Autodesk Inventor part; units mm, degrees
ref_plane "YZ Plane" through (0, 0, 0) normal (1, 0, 0) x (0, 1, 0)
ref_plane "XZ Plane" through (0, 0, 0) normal (0, 1, 0) x (-1, 0, 0)
ref_plane "XY Plane" through (0, 0, 0) normal (0, 0, 1) x (1, 0, 0)
sketch "Sketch1" plane through (0, 0, 0) normal (0, 0, 1) x (1, 0, 0)
  line L0 (2.1516, 4.7552) -> (14.9532, 4.7552)
  line L1 (14.9532, 4.7552) -> (14.9532, -2.1028)
  line L2 (14.9532, -2.1028) -> (2.1516, -2.1028)
  line L3 (2.1516, -2.1028) -> (2.1516, 4.7552)
  point P0 (0, 0)
  dimension "d0" = 12.8016
  dimension "d1" = 6.858
extrude "Extrusion1" add sketch "Sketch1" along normal blind 13.7414
sketch "Sketch2" plane through (0, 0, 13.7414) normal (0, 0, 1) x (1, 0, 0)
  circle A0 centre (8.5524, 1.3262) radius 2.921
  line L0 (14.9532, -2.1028) -> (14.9532, 4.7552)
  line L1 (14.9532, 4.7552) -> (2.1516, 4.7552)
  point P0 (0, 0)
  dimension "d4" = 5.842
  dimension "d5" = 6.4008
  dimension "d6" = 3.429
extrude "Extrusion2" add sketch "Sketch2" along normal blind 8.89
sketch "Sketch3" plane through (8.5524, 1.3262, 22.6314) normal (0, 0, 1) x (1, 0, 0)
  circle A0 centre (0, 0) radius 1.4986
  point P0 (-8.5524, -1.3262)
  dimension "d9" = 2.9972
extrude "Extrusion3" add sketch "Sketch3" along normal blind 9.906
properties part number "Switch"
Geometry: final body of the model. Coordinates: model frame, mm. A direction names the side the tool comes from. Give positions to 0.01 mm unless a question says otherwise; leave off trailing zeros. Write each loop counter-clockwise with the first axis right and the second up, starting at its lowest first coordinate (ties: lowest second). Pieces come first, ordered by that corner, then holes. Notation, with made-up numbers: M 50.5,73 L 109.5,73 A25 ccw 109.5,112 Z; hole C 43.5,-8 d6. An arc over 180 degrees is marked long. Answer in a Markdown table with one row per item. Add a question column.
(1) Section A-A on x = 13.25. Return loops of the section in (y, z).
(2) Reachability of faces 1 (the flat face through (2.152, 1, 7)), 2 (the flat face through (8, 3, 22.631)) from +Z, -Z, +X, -X, +Y, -Y: full face, straight path, thin tool, end or side. Return the list, or none.
(3) Section B-B on y = 2. Return loops of the section in (x, z), and give its area (3 significant figures).
(4) Section C-C on x = 8.5. Return loops of the section in (y, z), and give its area (3 significant figures).
(5) Section D-D on z = 24.5. Return loops of the section in (x, y), and give its area (3 significant figures).
(6) Ray query, line 1 (Z direction, x = 7, y = 1.5); line 2 (Z direction, x = 5.5, y = -1); line 3 (Y direction, x = 7.5, z = 14). Return the intervals inside material, ascending.
(7) First-contact query: pin 1 (3 mm diameter, centred on x = 8.5, z = 16, fed in from +Y). Flat tip, straight axial feed; report the tip coordinate or a pass-through.
Result set:
| question | item | result |
|---|---|---|
| 1 | outline | M -2.1,0 L 4.76,0 L 4.76,13.74 L -2.1,13.74 Z |
| 2 | face 1 | +Z, -Z, -X, +Y, -Y |
| 2 | face 2 | +Z |
| 3 | outline | M 2.15,0 L 14.95,0 L 14.95,13.74 L 11.39,13.74 L 11.39,22.63 L 9.89,22.63 L 9.89,32.54 L 7.21,32.54 L 7.21,22.63 L 5.71,22.63 L 5.71,13.74 L 2.15,13.74 Z |
| 3 | area | 253 mm^2 |
| 4 | outline | M -2.1,0 L 4.76,0 L 4.76,13.74 L 4.25,13.74 L 4.25,22.63 L 2.82,22.63 L 2.82,32.54 L -0.17,32.54 L -0.17,22.63 L -1.59,22.63 L -1.59,13.74 L -2.1,13.74 Z |
| 4 | area | 176 mm^2 |
| 5 | outline | C 8.55,1.33 d3 |
| 5 | area | 7.06 mm^2 |
| 6 | line 1 | z = 0 to 22.63 |
| 6 | line 2 | z = 0 to 13.74 |
| 6 | line 3 | y = -1.4 to 4.05 |
| 7 | pin 1 | stops at y = 4.25 |
